The model under review builds one solid part; all positions refer to its coordinate system, in mm. A direction names the side the tool comes from. Coordinates: 2 decimals unless noted, no trailing zeros. Write each loop counter-clockwise with the first axis right and the second up, starting at its lowest first coordinate (ties: lowest second). Pieces come first, ordered by that corner, then holes.
1) Add section B-B, the plane y = 0. State the section outline as (x, z) points.
2) Add section C-C, the plane z = -2.5. State the section outline as (x, y) points.
3) For P1, Ø5, axis at x = -7.75, y = -13.42, coming from the +Z side; P2, Ø5, axis at x = -12.5, z = -27.5, coming from the +Y side; P3, Ø3.5, axis at x = -0.5, z = 17.5, coming from the +Y side, all flat-tipped, find the tip position at first contact; note any pin that passes through.
4) For line 1 (Y direction, x = 7.75, z = -7.25); line 2 (Y direction, x = 7, z = -2); line 3 (Z direction, x = -10, y = 0.5), list the stretches that pass through material, from the lowest coordinate up.
5) Mouldability with a two-part tool opening along Y and no side actions: class faces 1 (the cylindrical face through (-4.01, -18.06, -14.3)), 2 (the flat face through (-8, 13, -10)), 3 (the flat face through (-0.1, -16.4, -29)) as released by +Y, released by -Y, zero draft, split by the parting line, or undercut.
6) Machinability: for faces 4 (the flat face through (0, 0, -58)), 5 (the cylindrical face through (6.644, 14.437, -4.93)), 6 (the flat face through (0, 9.5, 16)), 7 (the cylindrical face through (-15.5, -4.88, -43.3)), which of the approach directions +Z, -Z, +X, -X, +Y, -Y give a long, thin tool a straight path to every point of the face, cutting with its end or side? Answer none if there is none.
7) Add section D-D, the plane z = -19. State the section outline as (x, y) points, then the cut area to 3 significant figures.
8) Add section A-A, the plane x = 0. State the section outline as (y, z) points.
Autodesk Inventor part; units mm, degrees
ref_plane "YZ Plane" through (0, 0, 0) normal (1, 0, 0) x (0, 1, 0)
ref_plane "XZ Plane" through (0, 0, 0) normal (0, 1, 0) x (-1, 0, 0)
ref_plane "XY Plane" through (0, 0, 0) normal (0, 0, 1) x (1, 0, 0)
sketch "Sketch1" plane through (0, 0, 0) normal (0, 0, 1) x (1, 0, 0)
  circle A0 centre (0, 0) radius 18.5
  line L0 (0, 0) -> (0, 7) construction
  circle A1 centre (0, 7) radius 6
  dimension "d0" = 37
  dimension "d1" = 7
  dimension "d2" = 12
extrude "Extrusion1" add sketch "Sketch1" against normal blind 29 contours A0 | A1
extrude "Extrusion2" add sketch "Sketch1" along normal blind 6 contours A1
sketch "Sketch2" plane through (0, 7, 6) normal (0, 0, 1) x (1, 0, 0)
  circle A0 centre (0, 0) radius 3
  point P0 (0, -7)
  dimension "d7" = 6
extrude "Extrusion3" add sketch "Sketch2" along normal blind 15.5
sketch "Sketch3" plane through (0, 0, -29) normal (0, 0, -1) x (-1, 0, 0)
  circle A0 centre (0, 0) radius 16.25
  dimension "d10" = 32.5
extrude "Extrusion4" add sketch "Sketch3" along normal blind 29
sketch "Sketch4" plane through (0, 7, 21.5) normal (0, 0, 1) x (1, 0, 0)
  circle A0 centre (0, 0) radius 3
  arc A1 (-1.6583, 2.5) -> (1.6583, 2.5) centre (0, 0) ccw
  line L0 (-4.0487, 2.5) -> (4.6782, 2.5)
  arc A2 (1.6583, 2.5) -> (-1.6583, 2.5) centre (0, 0) ccw
  point P0 (0, -7)
  point P1 (0, -3)
  point P2 (-1.6583, 2.5)
  point P3 (1.6583, 2.5)
  dimension "d13" = 6
  dimension "d14" = 5.5
extrude "Extrusion5" cut sketch "Sketch4" against normal blind 12 contours L0 A0 picked at (-0.1169, 2.6598)
sketch "Sketch5" plane through (0, 0, 0) normal (0, 0, 1) x (1, 0, 0)
  circle A0 centre (0, 0) radius 15.5 construction
  line L0 (-7.75, -13.4234) -> (12.777, 22.1304) construction
  line L1 (0, 0) -> (25.5539, 0) construction
  line L2 (7.75, -13.4234) -> (-11.3824, 19.7148) construction
  line L3 (0, 0) -> (22.7647, 0) construction
  circle A1 centre (-15.5, 0) radius 1.5
  circle A2 centre (-7.75, 13.4234) radius 1.5
  circle A3 centre (7.75, 13.4234) radius 1.5
  circle A4 centre (15.5, 0) radius 1.5
  circle A5 centre (7.75, -13.4234) radius 1.5
  circle A6 centre (-7.75, -13.4234) radius 1.5
  dimension "d17" = 31
  dimension "d18" = 60
  dimension "d19" = 120
  dimension "d20" = 3
  dimension "d21" = 3
  dimension "d22" = 3
  dimension "d23" = 3
  dimension "d24" = 3
  dimension "d25" = 3
extrude "Extrusion6" cut sketch "Sketch5" against normal blind 10
properties part number "motor12kg"
Geometry results:
1. outline: (-18.5, -29) - (-16.25, -29) - (-16.25, -58) - (16.25, -58) - (16.25, -29) - (18.5, -29) - (18.5, 0) - (17, 0) - (17, -10) - (14, -10) - (14, 0) - (-14, 0) - (-14, -10) - (-17, -10) - (-17, 0) - (-18.5, 0) - close
2. outline: circle Ø37 at (0, 0); hole circle Ø3 at (-15.5, 0); hole circle Ø3 at (-7.75, -13.42); hole circle Ø3 at (-7.75, 13.42); hole circle Ø3 at (7.75, -13.42); hole circle Ø3 at (7.75, 13.42); hole circle Ø3 at (15.5, 0)
3. P1: stops at z = 0
3. P2: stops at y = 15.56
3. P3: stops at y = 9.5
4. line 1: y = -16.8 to -14.92, -11.92 to 11.92, 14.92 to 16.8
4. line 2: y = -17.12 to -14.72, -12.12 to 12.12, 14.72 to 17.12
4. line 3: z = -58 to 0
5. face 1: split by the parting line
5. face 2: undercut
5. face 3: zero draft
6. face 4: -Z, +X, -X, +Y, -Y
6. face 5: +Z
6. face 6: +Z, +X, -X, +Y
6. face 7: -Z
7. outline: circle Ø37 at (0, 0)
7. area: 1,080 mm2
8. outline: (-18.5, -29) - (-16.25, -29) - (-16.25, -58) - (16.25, -58) - (16.25, -29) - (18.5, -29) - (18.5, 0) - (13, 0) - (13, 6) - (10, 6) - (10, 9.5) - (9.5, 9.5) - (9.5, 21.5) - (4, 21.5) - (4, 6) - (1, 6) - (1, 0) - (-18.5, 0) - close
